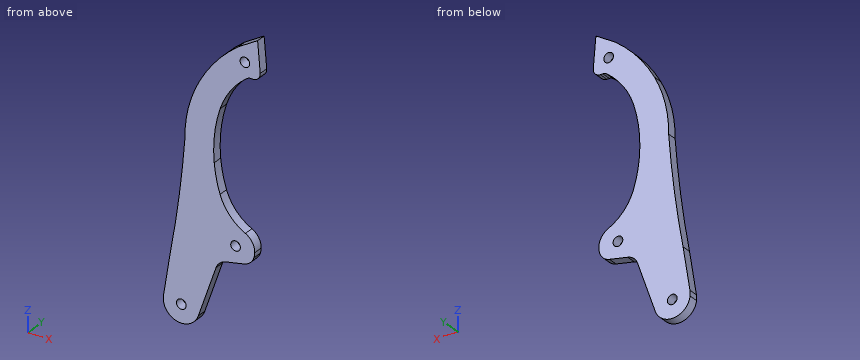
Autodesk Inventor part; units mm, degrees
ref_plane "YZ Plane" through (0, 0, 0) normal (1, 0, 0) x (0, 1, 0)
ref_plane "XZ Plane" through (0, 0, 0) normal (0, 1, 0) x (-1, 0, 0)
ref_plane "XY Plane" through (0, 0, 0) normal (0, 0, 1) x (1, 0, 0)
sketch "Sketch4" plane through (0, 0, 0) normal (0, 1, 0) x (-1, 0, 0)
  arc A0 (8.5248, -5.2299) -> (8.4715, -3.5145) centre (2.5627, -4.5564) ccw
  circle A1 centre (-13.8365, 17.7403) radius 1.5
  circle A2 centre (2.9812, -4.5435) radius 1.5
  arc A3 (-18.1395, 21.8135) -> (-18.0355, 13.56) centre (-13.8365, 17.7403) ccw
  arc A4 (-9.0304, 31.4366) -> (-7.2225, 40.1949) centre (-45.2058, 43.4695) ccw
  arc A5 (-18.1395, 21.8135) -> (-9.0304, 31.4366) centre (-23.8893, 36.3791) ccw
  line L0 (6.3335, 9.9302) -> (8.4977, -3.6654)
  circle A6 centre (-16.5155, 72.4101) radius 3.2
  line L1 (-20.6719, 80.2448) -> (-14.7774, 76.6686)
  arc A7 (-2.5338, 62.5638) -> (-14.7774, 76.6686) centre (-39.7178, 42.6529) ccw
  arc A8 (1.8655, 44.4721) -> (-2.5338, 62.5638) centre (-35.3105, 45.0128) ccw
  arc A9 (1.8655, 44.4721) -> (6.3335, 9.9302) centre (325.703, 68.8005) ccw
  line L2 (-21.6848, 68.4625) -> (-20.6719, 80.2448)
  line L3 (-18.8545, 68.4625) -> (-21.6848, 68.4625)
  line L4 (-18.8545, 68.4625) -> (-17.8545, 68.4625)
  arc A10 (-9.0296, 56.61) -> (-17.8545, 68.4625) centre (-31.443, 49.1333) ccw
  arc A11 (-7.2225, 40.1949) -> (-9.0296, 56.61) centre (-48.1916, 43.9919) ccw
  line L5 (-8.5324, 11.672) -> (-2.2983, -6.3679)
  line L6 (-8.5324, 11.672) -> (-18.0355, 13.56)
  arc A12 (8.4977, -3.6654) -> (8.4715, -3.5145) centre (2.9812, -4.5435) ccw
  arc A13 (-2.2983, -6.3679) -> (8.5248, -5.2299) centre (2.9812, -4.5435) ccw
  arc A14 (8.4977, -3.6654) -> (8.4715, -3.5145) centre (2.9812, -4.5435) ccw
  point P0 (0, 0)
  point P1 (-5.4967, 17.4778)
  point P2 (-7.3422, 22.2297)
  point P3 (-8.8923, 40.8853)
  point P4 (7.4044, -1.132)
  point P5 (0, 0)
  dimension "d11" = 3
  dimension "d23" = 6.4
extrude "Extrusion4" add sketch "Sketch4" along normal blind 3 contours A13 L5 L6 A3 A5 A4 A11 A10 L4 L3 L2 L1 A7 A8 A9 L0 A0 | A6
fillet "Fillet5" radius 5.2 1 edges at (18.1395, 1.5, 21.8135)
fillet "Fillet6" radius 2 1 edges at (17.8545, 1.5, 68.4625)
fillet "Fillet8" radius 2.2 1 edges at (21.6848, 1.5, 68.4625)
sketch "Sketch7" plane through (0, 3, 0) normal (0, 1, 0) x (1, 0, 0)
  circle A0 centre (16.7249, -72.6774) radius 1.5
  dimension "d31" = 3
extrude "Extrusion7" cut sketch "Sketch7" against normal through all
fillet "Fillet9" radius 4 1 edges at (18.0355, 1.5, 13.56)
fillet "Fillet10" radius 4 1 edges at (8.5324, 1.5, 11.672)
properties part number "claw2" material "ABS Plastic"
Design review of the part built by this model. Coordinates are the model's own, in mm. Give positions to 0.01 mm unless a question says otherwise; leave off trailing zeros. Loops run counter-clockwise (first coordinate to the right, second up) from the corner with the lowest first, then second, coordinate; pieces in that order, holes last. Notation, with made-up numbers: M 57.5,-22.5 L 113.5,-22.5 A33 ccw 113.5,16.5 Z; hole C 11.5,-9.75 d1. An arc over 180 degrees is marked long. One line per question, with ' | ' between items. Start each with the question number.
1. To check wall thickness, follow L1, parallel to Z at x = 13.5, y = 2.85; L2, parallel to Z at x = 17.5, y = 2.95; L3, parallel to Z at x = 10.5, y = 1.2. State the ranges of each line that lie inside material, in increasing order.
2. Add section B-B (x = 0.5). Write out the cut boundary in (y, z), plus the area to 3 significant figures.
3. Add section C-C (z = 23.5). Write out the cut boundary in (x, y), plus the area to 3 significant figures.
4. Insertion check: P1, Ø1.5, axis at y = 2.5, z = 2.5, coming from the -X side; P2, Ø8, axis at x = 1.5, z = 13.5, coming from the -Y side. Each pin has a flat end and moves straight along its axis. Give the tip position at first contact, or say it passes through.
5. Add section A-A (y = 2.45). Give the number of separate pieces and of enclosed holes in the cut face, plus the area to 3 significant figures.
Worked out:
1) L1: z = 12.66 to 16.28, 19.2 to 24.66, 64.51 to 75.69 | L2: z = 13.61 to 22.01, 68.19 to 71.39, 73.96 to 78.32 | L3: z = 12.05 to 28.26, 60.07 to 73.07
2) outline: M 0,-8.91 L 3,-8.91 L 3,58.07 L 0,58.07 Z | area: 201 mm²
3) outline: M -4.13,0 L 14.98,0 L 14.98,3 L -4.13,3 Z | area: 57.3 mm²
4) P1: stops at x = -7.64 | P2: stops at y = 0
5) separate pieces: 1 | enclosed holes: 3 | area: 1,090 mm²
